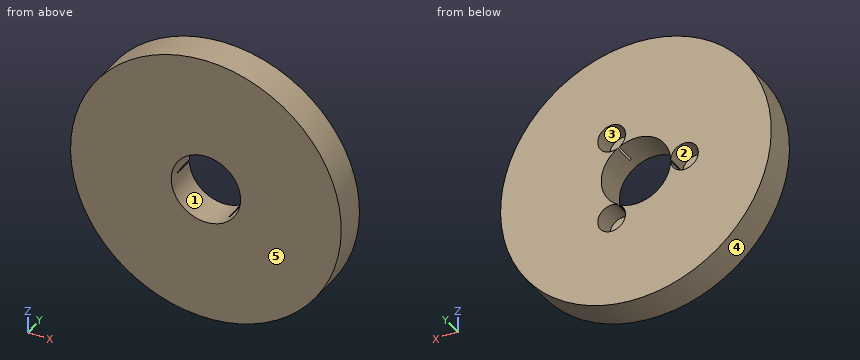
```python
from build123d import *

# Parameters (mm, degrees)
SKETCH1_R           = 97.5
BOSS_EXTRUDE1_DEPTH = 24
SKETCH2_R           = 25
CUT_EXTRUDE1_DEPTH  = 140.958922545
SKETCH3_R           = 10
CUT_EXTRUDE2_DEPTH  = 15.823761
CIRPATTERN1_START   = 8.176238575
CIRPATTERN1_DEPTH   = 15.823761425


# Read off the part's stored shape, not the designer's step: CirPattern1
with BuildPart() as part:
    # Sketch1 → Boss-Extrude1 (new body)
    with BuildSketch(Plane(origin=(0, 0, 0), x_dir=(1, 0, 0), z_dir=(0, 1, 0))):
        with Locations(Location((0, 0, 0), (0, 0, 270))):
            Circle(SKETCH1_R)
    extrude(amount=BOSS_EXTRUDE1_DEPTH)

    # Sketch2 → Cut-Extrude1 (cut, through all)
    with BuildSketch(Plane(origin=(0, 0, 0), x_dir=(1, 0, 0), z_dir=(0, 1, 0))):
        with Locations(Location((0, 0, 0), (0, 0, 270))):
            Circle(SKETCH2_R)
    extrude(amount=CUT_EXTRUDE1_DEPTH, mode=Mode.SUBTRACT)

    # Sketch3 → Cut-Extrude2 (cut)
    with BuildSketch(Plane(origin=(0, 24, 0), x_dir=(1, 0, 0), z_dir=(0, 1, 0))):
        with Locations((-34.969247783, 0)):
            Circle(SKETCH3_R)
    extrude(amount=-CUT_EXTRUDE2_DEPTH, mode=Mode.SUBTRACT)

    # CirPattern1 outline → CirPattern1 (cut)
    with BuildSketch(Plane(origin=(0, 0, 0), x_dir=(1, 0, 0), z_dir=(0, 1, 0)).offset(CIRPATTERN1_START)):
        with BuildLine():
            ThreePointArc((11.921838951, 21.974297623), (12.5, 21.650635094), (13.069380497, 21.311764203))
            ThreePointArc((13.069380497, 21.311764203), (22.484623886, 38.944510972), (11.921838951, 21.974297623))
        make_face()
        with BuildLine():
            ThreePointArc((13.069380497, -21.311764203), (12.5, -21.650635094), (11.921838951, -21.974297623))
            ThreePointArc((11.921838951, -21.974297623), (22.484623886, -38.944510972), (13.069380497, -21.311764203))
        make_face()
    extrude(amount=CIRPATTERN1_DEPTH, mode=Mode.SUBTRACT)


solid = part.part
```
Input: part model. Units: mm. Frame: model coordinates. Face numbers are marked on the shaded views. A direction names the side the tool comes from. Coordinates: 2 decimals unless noted, no trailing zeros. Loops run counter-clockwise (first coordinate to the right, second up) from the corner with the lowest first, then second, coordinate; pieces in that order, holes last. Notation, with made-up numbers: M 3.25,44 L 18.25,44 A24 cw 18.25,71 Z; hole C -25,77.25 d9. An arc over 180 degrees is marked long. Use a Markdown table: item, result. Add a question column.
1) Draft query along Z for the marked faces 3, 4 and 5. Return one class per face: +Z half, -Z half, draft (parallel to the pull), parting line (faces both ways), or undercut.
2) Section C-C, the plane y = 3.5. Return the cut outline in (x, z).
3) Section D-D, the plane x = 31. Return the cut outline in (y, z).
4) Line query: L1, parallel to Z at x = 14, y = 12.75; L2, parallel to Y at x = 10, z = 27.5; L3, parallel to Z at x = -21.5, y = 17.5. Output: solid intervals per line, ascending. Write a range as from..to.
5) Section A-A, the plane x = 0. Return the cut outline in (y, z).
6) Section B-B, the plane z = -17. Return the cut outline in (x, y).
7) Set-up query: the marked faces 1 and 2. Return all of +Z, -Z, +X, -X, +Y, -Y with unobstructed straight access to the full face (end or side cutting, diameter ignored); none if empty.
8) Pin query (flat end, axial travel): P1, Ø1, axis at y = 5.5, z = 74.5, coming from the -X side; P2, Ø10, axis at y = 16.5, z = -16.5, coming from the +X side; P3, Ø1, axis at x = -8, z = 63, coming from the -Y side; P4, Ø6, axis at x = 14.5, z = 34, coming from the +Y side. Return the tip coordinate at first contact, or that it passes through.
Answer below:
| question | item | result |
|---|---|---|
| 1 | face 3 | undercut |
| 1 | face 4 | parting line |
| 1 | face 5 | draft |
| 2 | outline | C 0,0 d195; hole C 0,0 d50 |
| 3 | outline | M 0,-92.44 L 24,-92.44 L 24,92.44 L 0,92.44 Z |
| 4 | L1 | -96.49..-39.66, -20.91..-20.71, 20.71..20.91, 39.66..96.49 |
| 4 | L2 | 0..8.18 |
| 4 | L3 | -95.1..-12.76, 12.76..95.1 |
| 5 | outline | M 0,-97.5 L 24,-97.5 L 24,-25 L 0,-25 Z; M 0,25 L 24,25 L 24,97.5 L 0,97.5 Z |
| 6 | outline | M -96.01,0 L -18.33,0 L -18.33,24 L -96.01,24 Z; M 18.33,0 L 96.01,0 L 96.01,24 L 18.33,24 Z |
| 7 | face 1 | +Y, -Y |
| 7 | face 2 | +Y |
| 8 | P1 | x = -63.48 |
| 8 | P2 | x = 96.82 |
| 8 | P3 | y = 0 |
| 8 | P4 | y = 8.18 |
